Part model, mm, in its own coordinate system. Face numbers are marked on the shaded views. A direction names the side the tool comes from. Round coordinates to 2 decimals unless told otherwise and drop trailing zeros. Write each loop counter-clockwise with the first axis right and the second up, starting at its lowest first coordinate (ties: lowest second). Pieces come first, ordered by that corner, then holes.
1) Saw through at B-B on z = 4.5. Write the cut outline in (x, y).
2) Drill centre lines: L1, parallel to Z at x = -2.75, y = -4.75; L2, parallel to X at y = -0.5, z = 7.5; L3, parallel to Y at x = -1.75, z = 6.25. Where is each one in solid material? Low to high.
3) Which spindle directions (+Z, -Z, +X, -X, +Y, -Y) get a long thin tool onto all of the face, cutting with end or side? Do the marked faces 1, 2, 3, 4 and 5. Say none if no direction does.
4) Saw through at C-C on y = -2.25. Write the cut outline in (x, z), and give its area (3 significant figures).
5) Flat gauge pins, fed straight in: pin 1 (1 mm diameter, centred on x = -5.5, z = 3, fed in from -Y); pin 2 (4 mm diameter, centred on y = 1, z = 8, fed in from +X); pin 3 (4 mm diameter, centred on x = -0.5, z = 7, fed in from -Y). Where does each tip first touch, or does it go through?
6) Saw through at D-D on x = -1. Write the cut outline in (y, z).
7) Pull direction Z, two halves, no side cores. Call the marked faces 6, 7, 8 and 9: +Z half, -Z half, draft (parallel to the pull), parting line (faces both ways), or undercut.
8) Saw through at A-A on x = -4.5. Write the cut outline in (y, z), and give its area (3 significant figures).
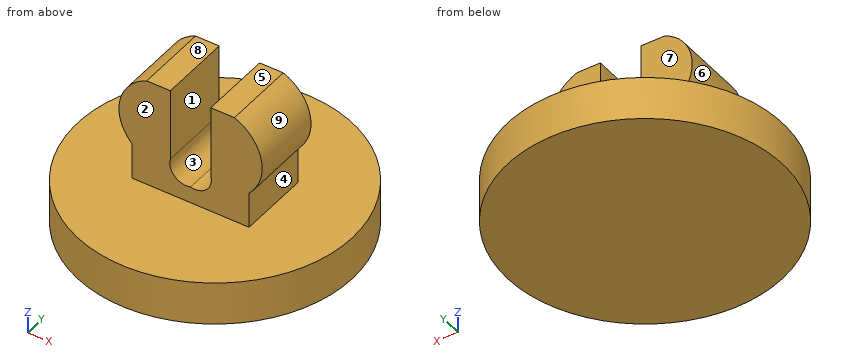
```python
from build123d import *

# Parameters (mm, degrees)
SKETCH1_R           = 9.5
BOSS_EXTRUDE1_DEPTH = 3
BOSS_EXTRUDE2_DEPTH = 2.5


with BuildPart() as part:
    # Sketch1 → Boss-Extrude1 (new body)
    with BuildSketch(Plane.XY):
        Circle(SKETCH1_R)
    extrude(amount=BOSS_EXTRUDE1_DEPTH)

    # Sketch3 → Boss-Extrude2 (add, symmetric)
    with BuildSketch(Plane(origin=(0, 0, 0), x_dir=(1, 0, 0), z_dir=(0, 1, 0))):
        with BuildLine():
            Line((-4.053033857, -5.5), (-4.053033857, -3))
            Line((-4.053033857, -3), (4.053033857, -3))
            Line((4.053033857, -3), (4.053033857, -5.5))
            ThreePointArc((4.053033857, -5.5), (4.899562702, -8.305363596), (3.036123017, -10.566838454))
            Line((3.036123017, -10.566838454), (1.4, -10.566838454))
            Line((1.4, -10.566838454), (1.4, -5.566838454))
            ThreePointArc((1.4, -5.566838454), (1.111291087, -4.450394141), (0, -4.142444699))
            ThreePointArc((0, -4.142444699), (-1.111291087, -4.450394141), (-1.4, -5.566838454))
            Line((-1.4, -5.566838454), (-1.4, -10.566838454))
            Line((-1.4, -10.566838454), (-3.036123017, -10.566838454))
            ThreePointArc((-3.036123017, -10.566838454), (-4.899562702, -8.305363596), (-4.053033857, -5.5))
        make_face()
    extrude(amount=BOSS_EXTRUDE2_DEPTH, both=True)


solid = part.part
```
Completed:
1. outline: (-4.05, -2.5) - (-1.16, -2.5) - (-1.16, 2.5) - (-4.05, 2.5) - close; (1.16, -2.5) - (4.05, -2.5) - (4.05, 2.5) - (1.16, 2.5) - close
2. L1: z = 0 to 3
2. L2: x = -4.95 to -1.4, 1.4 to 4.95
2. L3: y = -2.5 to 2.5
3. face 1: +Z, +Y, -Y
3. face 2: +Z, +X, -X, -Y
3. face 3: +Y, -Y
3. face 4: +X, +Y, -Y
3. face 5: +Z, +X, -X, +Y, -Y
4. outline: (-9.23, 0) - (9.23, 0) - (9.23, 3) - (4.05, 3) - (4.05, 5.5) arc R3.11 ccw to (3.04, 10.57) - (1.4, 10.57) - (1.4, 5.57) arc R1.15 cw to (0, 4.14) arc R1.15 cw to (-1.4, 5.57) - (-1.4, 10.57) - (-3.04, 10.57) arc R3.11 ccw to (-4.05, 5.5) - (-4.05, 3) - (-9.23, 3) - close
4. area: 104 mm2
5. pin 1: stops at y = -8.08
5. pin 2: stops at x = 4.96
5. pin 3: stops at y = -2.5
6. outline: (-9.45, 0) - (9.45, 0) - (9.45, 3) - (2.5, 3) - (2.5, 4.35) - (-2.5, 4.35) - (-2.5, 3) - (-9.45, 3) - close
7. face 6: undercut
7. face 7: draft
7. face 8: +Z half
7. face 9: undercut
8. outline: (-8.37, 0) - (8.37, 0) - (8.37, 3) - (-8.37, 3) - close; (-2.5, 6.07) - (2.5, 6.07) - (2.5, 9.32) - (-2.5, 9.32) - close
8. area: 66.5 mm2
